Could you check a few things on this model? Use its own coordinates, in mm. A direction names the side the tool comes from. Round coordinates to 2 decimals unless told otherwise and drop trailing zeros. Write each loop counter-clockwise with the first axis right and the second up, starting at its lowest first coordinate (ties: lowest second). Pieces come first, ordered by that corner, then holes.
```python
from build123d import *

# Parameters (mm, degrees)
BOSS_EXTRUDE1_DEPTH = 38.1
BOSS_EXTRUDE2_DEPTH = 47.625
BOSS_EXTRUDE3_DEPTH = 3.175
FILLET1_R           = 1.5875
FILLET2_R           = 0.79375


with BuildPart() as part:
    # Sketch1 → Boss-Extrude1 (new body)
    with BuildSketch(Plane(origin=(0, 0, 0), x_dir=(1, 0, 0), z_dir=(0, 1, 0))):
        Polygon((0, 0), (0, -34.925), (26.9875, -34.925), (26.9875, -25.4), (23.8125, -25.4), (23.8125, -31.75), (3.175, -31.75), (3.175, 0), align=None)
    extrude(amount=BOSS_EXTRUDE1_DEPTH)

    # Sketch2 → Boss-Extrude2 (add)
    with BuildSketch(Plane.XY.offset(34.925)):
        with BuildLine():
            Line((0, 19.05), (0, 0))
            Line((0, 0), (26.9875, 0))
            Line((26.9875, 0), (26.9875, 19.05))
            ThreePointArc((26.9875, 19.05), (13.49375, 25.4), (0, 19.05))
        make_face()
    extrude(amount=BOSS_EXTRUDE2_DEPTH)

    # Sketch3 → Boss-Extrude3 (add)
    with BuildSketch(Plane.XY.offset(82.55)):
        with BuildLine():
            Line((0, 19.05), (0, 23.56829895))
            ThreePointArc((0, 23.56829895), (13.49375, 28.575), (26.9875, 23.56829895))
            Line((26.9875, 23.56829895), (26.9875, 19.05))
            Line((26.9875, 19.05), (26.9875, 0))
            Line((26.9875, 0), (0, 0))
            Line((0, 0), (0, 19.05))
        make_face()
    extrude(amount=BOSS_EXTRUDE3_DEPTH)

    # Fillet1
    fillet1_edges = [part.edges().sort_by_distance(p)[0] for p in [
        (13.49375, 38.1, 34.925),
        (0, 0, 42.8625),
        (1.5875, 0, 0),
        (26.9875, 38.1, 30.1625),
        (26.9875, 19.05, 25.4),
        (26.9875, 28.575, 34.925),
        (0, 28.575, 34.925),
        (0, 19.05, 0),
        (25.4, 38.1, 25.4),
        (26.9875, 11.784149475, 85.725),
        (13.49375, 28.575, 85.725),
        (0, 11.784149475, 85.725),
        (13.49375, 0, 85.725),
        (1.5875, 38.1, 0),
        (0, 38.1, 17.4625),
        (25.4, 0, 25.4),
        (26.9875, 0, 55.5625),
    ]]
    fillet(fillet1_edges, radius=FILLET1_R)

    # Fillet2
    fillet2_edges = [part.edges().sort_by_distance(p)[0] for p in [
        (26.9875, 21.309149475, 82.55),
        (13.49375, 28.575, 82.55),
        (0, 21.309149475, 82.55),
    ]]
    fillet(fillet2_edges, radius=FILLET2_R)


solid = part.part
```
Q1. We'd pull the mould along Z, two halves only. Please class faces 1 (the flat face through (3, 38.1, 23)), 2 (the flat face through (14, 26, 82.55)), 3 (the cylindrical face through (24.6, 0.45, 25.88)): pulls with the +Z half, pulls with the -Z half, needs draft (parallel to the pull), parting line crosses it, or undercut.
Q2. If I drill on L1, parallel to Z at x = 15.25, y = 12 (3 decimals); L2, parallel to X at y = 24.5, z = 23.5 (3 decimals); L3, parallel to Z at x = 9, y = 32.5 (3 decimals), over which ranges is the centre line in solid material (lowest first)?
Q3. I'm going to push flat-ended pins straight in: pin 1 Ø1 at (x, z) = (8, 41) entering from +Y; pin 2 Ø16 at (y, z) = (22, 9) entering from +X (3 decimals); pin 3 Ø2 at (x, y) = (7.5, 25) entering from -Z. Where does each tip first touch, or does it pass through?
Q4. On a 3-axis mill with a long thin cutter (end or side, diameter ignored), from which of +Z, -Z, +X, -X, +Y, -Y can I reach the whole of each face in a straight line? I mean faces 4 (the flat face through (14, 19, 31.75)), 5 (the flat face through (25, 19, 25.4)), 6 (the cylindrical face through (24.6, 37.62, 25.85)), 7 (the cylindrical face through (13.7, 25.4, 58)), 8 (the cylindrical face through (13.288, 28.574, 83.735)). Say none if no direction works.
Q5. Imagine slicing it at C-C, the plane z = 14. Write out the boundary of the cut face in (x, y) (1 decimal), then the cut area to 3 significant figures.
Results found:
1. face 1: needs draft
1. face 2: undercut
1. face 3: pulls with the -Z half
2. L1: z = 31.75 to 85.725
2. L2: x = 0 to 3.175
2. L3: z = 31.75 to 34.925
3. pin 1: stops at y = 24.67
3. pin 2: stops at x = 3.175
3. pin 3: stops at z = 31.75
4. face 4: -Z, +Y, -Y
4. face 5: -Z, +X, +Y, -Y
4. face 6: -Z, +X, +Y
4. face 7: +Y
4. face 8: +Z, +Y
5. outline: (0, 1.6) arc R1.6 ccw to (1.6, 0) - (3.2, 0) - (3.2, 38.1) - (1.6, 38.1) arc R1.6 ccw to (0, 36.5) - close
5. area: 120 mm2
